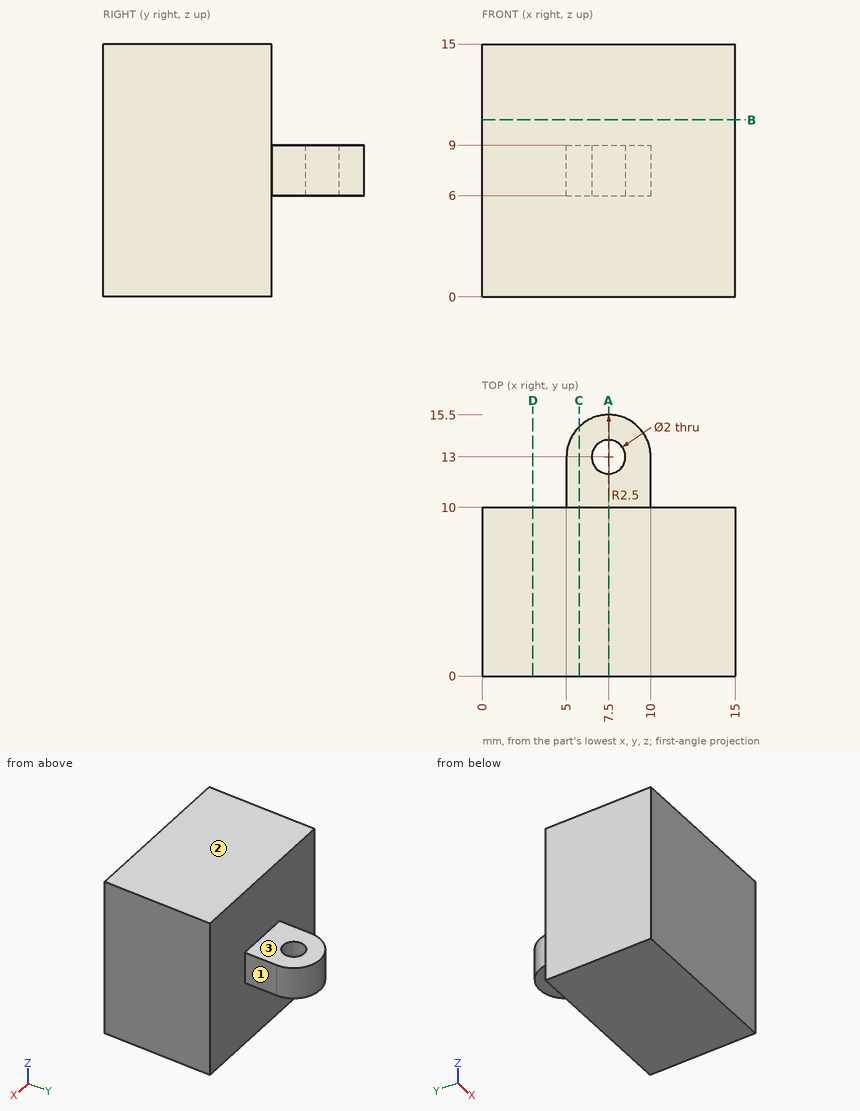
Verification items for this drawing (mm, ordinates from the low corner). A direction names the side the tool comes from. Give positions to 0.01 mm unless a question says otherwise; leave off trailing zeros. Loops run counter-clockwise (first coordinate to the right, second up) from the corner with the lowest first, then second, coordinate; pieces in that order, holes last. Notation, with made-up numbers: M -4.75,3.5 L 39.25,3.5 A34 cw 39.25,37.5 Z; hole C -18.75,-32 d6. An arc over 180 degrees is marked long. Write item = value, one per line.
(1) Sectioned sample at B-B, the plane z = 10.5. Record the cut outline in (x, y), plus the area to 3 significant figures.
Answer below:
outline = M 0,0 L 15,0 L 15,10 L 0,10 Z
area = 150 mm2
(2) Sectioned sample at A-A, the plane x = 7.5. Record the cut outline in (y, z), plus the area to 4 significant figures.
Answer below:
outline = M 0,0 L 10,0 L 10,6 L 12,6 L 12,9 L 10,9 L 10,15 L 0,15 Z; M 14,6 L 15.5,6 L 15.5,9 L 14,9 Z
area = 160.5 mm2
(3) Sectioned sample at C-C, the plane x = 5.75. Record the cut outline in (y, z), plus the area to 3 significant figures.
Answer below:
outline = M 0,0 L 10,0 L 10,6 L 14.79,6 L 14.79,9 L 10,9 L 10,15 L 0,15 Z
area = 164 mm2
(4) Tool access check on the marked faces 1, 2 and 3. Record the directions out of +Z, -Z, +X, -X, +Y, -Y that give a thin tool (end or side, any length) a straight path to the whole face; none if there is none.
Answer below:
face_1 = +Z, -Z, +X, +Y
face_2 = +Z, +X, -X, +Y, -Y
face_3 = +Z, +X, -X, +Y
(5) Material ranges on line 1 (Y direction, x = 7.5, z = 7.55); line 2 (Y direction, x = 7, z = 2); line 3 (Z direction, x = 7.5, y = 14.25), recorded low to high. Write a range as [from, to].
Answer below:
line_1 = [0, 12], [14, 15.5]
line_2 = [0, 10]
line_3 = [6, 9]
(6) Gauge pin test, flat ends, axial feed: pin 1 Ø0.9 at (y, z) = (11.5, 8) entering from -X; pin 2 Ø1.5 at (y, z) = (5.5, 9) entering from -X; pin 3 Ø1.5 at (x, y) = (8.5, 13) entering from -Z; pin 4 Ø2 at (x, z) = (13.5, 11.5) entering from +Y. Record the tip position at first contact, or that the pin passes through.
Answer below:
pin_1 = 5
pin_2 = 0
pin_3 = 6
pin_4 = 10
(7) Sectioned sample at D-D, the plane x = 3. Record the cut outline in (y, z), plus the area to 3 significant figures.
Answer below:
outline = M 0,0 L 10,0 L 10,15 L 0,15 Z
area = 150 mm2
